Check sheet for the drawn part. Datum: minimum x, y, z corner. Units: mm. A direction names the side the tool comes from. Give positions to 0.01 mm unless a question says otherwise; leave off trailing zeros. Order: outer loops, then holes, each group sorted by start corner. A loop starts at its lowest first (then second) coordinate and runs counter-clockwise, first axis right, second up. Notation, with made-up numbers: (34.5, 54.25) -> (69.5, 54.25) arc R25 ccw to (69.5, 93.25) -> close; hole circle Ø6 at (89.25, -22). An arc over 180 degrees is marked (long way). Answer in a Markdown table with one row per item. Add a question column.
(1) Cross-section at D-D (y = 61). Record the cut outline in (x, z), then the cut area to 3 significant figures.
(2) Cross-section at A-A (x = 62). Record the cut outline in (y, z), then the cut area to 3 significant figures.
(3) Go/stop test with flat-tipped pins: pin 1 (5.5 mm diameter, centred on x = 72, z = 5, fed in from -Y); pin 2 (5 mm diameter, centred on x = 129.5, z = 4.5, fed in from +Y); pin 3 (8 mm diameter, centred on y = 46, z = 2.5, fed in from -X); pin 4 (4 mm diameter, centred on x = 48.5, y = 41.5, fed in from -Z). Record where each tip stops, or that it passes through.
(4) Set-up check for the marked faces 1, 2, 3, 4 and 5: record each of +Z, -Z, +X, -X, +Y, -Y from which the full face is reachable in a straight line by a thin tool's end or side.
(5) Thickness scan on L1, parallel to X at y = 18, z = 15.25; L2, parallel to Y at x = 62, z = 8.75; L3, parallel to Y at x = 63, z = 6.25. Record the ranges inside material, lowest first. Write a range as [from, to].
(6) Cross-section at C-C (y = 33.5). Record the cut outline in (x, z), then the cut area to 3 significant figures.
(7) Cross-section at B-B (z = 3.5). Record the cut outline in (x, y).
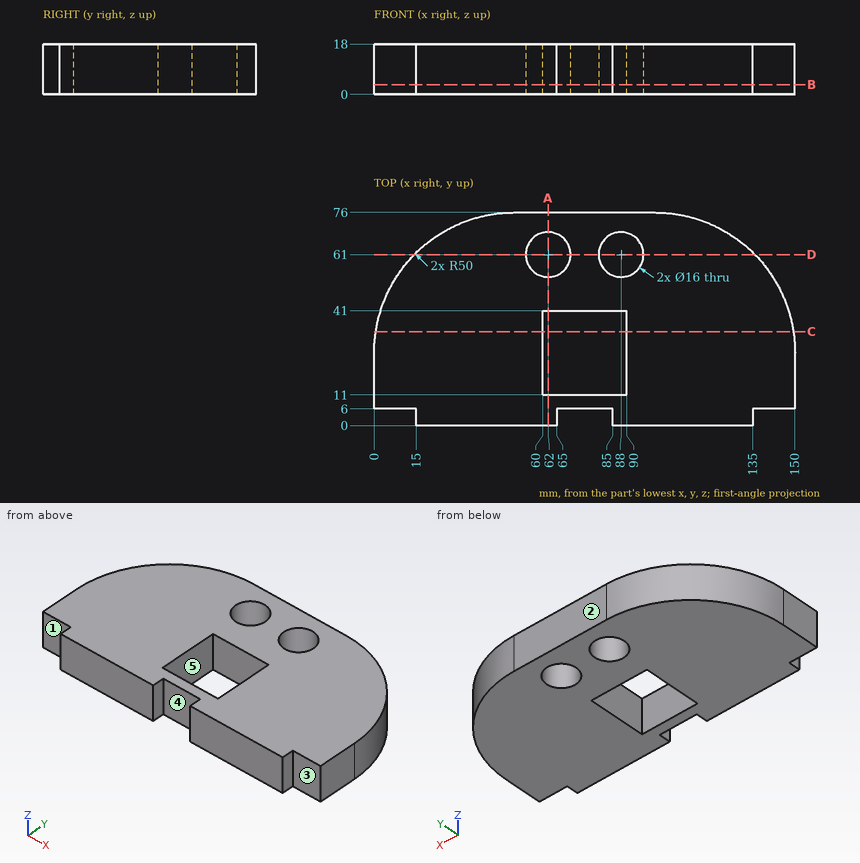
Answer below:
| question | item | result |
|---|---|---|
| 1 | outline | (14.29, 0) -> (54, 0) -> (54, 18) -> (14.29, 18) -> close; (70, 0) -> (80, 0) -> (80, 18) -> (70, 18) -> close; (96, 0) -> (135.71, 0) -> (135.71, 18) -> (96, 18) -> close |
| 1 | area | 1,610 mm² |
| 2 | outline | (0, 0) -> (11, 0) -> (11, 18) -> (0, 18) -> close; (41, 0) -> (53, 0) -> (53, 18) -> (41, 18) -> close; (69, 0) -> (76, 0) -> (76, 18) -> (69, 18) -> close |
| 2 | area | 540 mm² |
| 3 | pin 1 | stops at y = 6 |
| 3 | pin 2 | stops at y = 68.08 |
| 3 | pin 3 | stops at x = 2.63 |
| 3 | pin 4 | stops at z = 0 |
| 4 | face 1 | +Z, -Z, -X, -Y |
| 4 | face 2 | +Z, -Z, +X, -X, +Y |
| 4 | face 3 | +Z, -Z, +X, -Y |
| 4 | face 4 | +Z, -Z, -Y |
| 4 | face 5 | +Z, -Z |
| 5 | L1 | x = [0, 60], [90, 150] |
| 5 | L2 | y = [0, 11], [41, 53], [69, 76] |
| 5 | L3 | y = [0, 11], [41, 53.06], [68.94, 76] |
| 6 | outline | (0.57, 0) -> (60, 0) -> (60, 18) -> (0.57, 18) -> close; (90, 0) -> (149.43, 0) -> (149.43, 18) -> (90, 18) -> close |
| 6 | area | 2,140 mm² |
| 7 | outline | (0, 6) -> (15, 6) -> (15, 0) -> (65, 0) -> (65, 6) -> (85, 6) -> (85, 0) -> (135, 0) -> (135, 6) -> (150, 6) -> (150, 26) arc R50 ccw to (100, 76) -> (50, 76) arc R50 ccw to (0, 26) -> close; hole circle Ø16 at (62, 61); hole (60, 11) -> (90, 11) -> (90, 41) -> (60, 41) -> close; hole circle Ø16 at (88, 61) |
